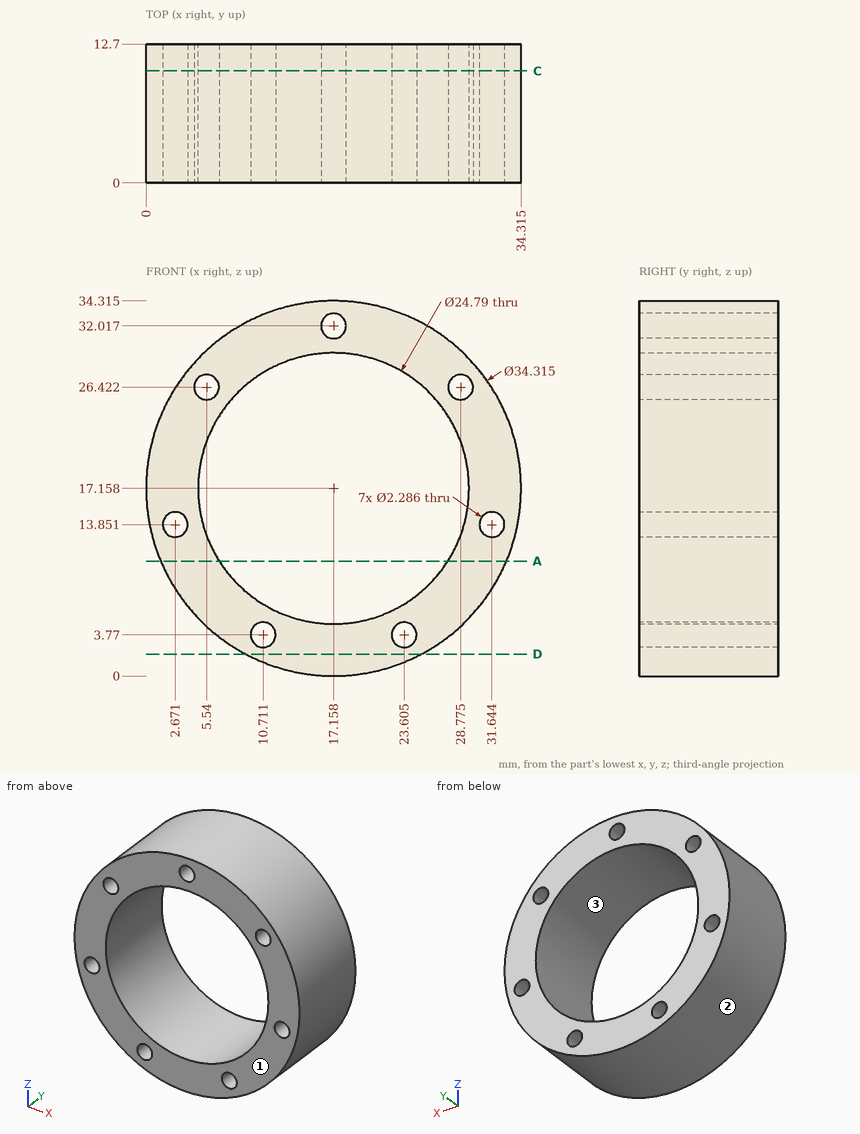
The drawing under review shows one solid part. Ordinate dimensions are in mm from its lowest x, y, z. Coordinates: 2 decimals unless noted, no trailing zeros. Loops run counter-clockwise (first coordinate to the right, second up) from the corner with the lowest first, then second, coordinate; pieces in that order, holes last. Notation, with made-up numbers: (42, 8.5) -> (54, 8.5) arc R19 cw to (54, 34.5) -> close; hole circle Ø6 at (65, -15.75). An arc over 180 degrees is marked (long way). Answer as a JSON object with one key per item and string values.
Q1. Take a section at C-C on y = 10.25. Give the number of separate pieces and of enclosed holes in the cut face.
Answer block:
{"separate pieces": "1", "enclosed holes": "8"}
Q2. Clearance check with flat-ended pins moving along their axes: pin 1 Ø4 at (x, y) = (13, 3.5) entering from +Z; pin 2 Ø5 at (x, y) = (6.5, 11) entering from +Z; pin 3 Ø3 at (x, y) = (5, 2.5) entering from +Z (1 decimal). State where each tip first meets the part, or that it passes through.
Answer block:
{"pin 1": "stops at z = 34.18", "pin 2": "stops at z = 32.25", "pin 3": "stops at z = 30.6"}
Q3. Take a section at D-D on z = 2. Give the boundary of the cut face in (x, y).
Answer block:
{"outline": "(9.12, 0) -> (25.2, 0) -> (25.2, 12.7) -> (9.12, 12.7) -> close"}
Q4. To check wall thickness, follow L1, parallel to Z at x = 15.5, y = 9.75 (1 decimal); L2, parallel to Z at x = 6.5, y = 9.25 (1 decimal). State the ranges of each line that lie inside material, in increasing order.
Answer block:
{"L1": "z = 0.1 to 4.9, 29.4 to 34.2", "L2": "z = 3.7 to 10.8, 23.5 to 25.8, 27 to 30.6"}
Q5. The part is to be moulded in two halves that separate along Z. For the marked faces 1, 2 and 3, say which applies: +Z half, -Z half, draft (parallel to the pull), parting line (faces both ways), or undercut.
Answer block:
{"face 1": "draft", "face 2": "parting line", "face 3": "undercut"}
Q6. Take a section at A-A on z = 10.5. Give the boundary of the cut face in (x, y) (1 decimal), plus the area to 3 significant figures.
Answer block:
{"outline": "(1.3, 0) -> (6.7, 0) -> (6.7, 12.7) -> (1.3, 12.7) -> close; (27.6, 0) -> (33, 0) -> (33, 12.7) -> (27.6, 12.7) -> close", "area": "136 mm^2"}
